Design review of the part shown in the three views and the two pictorial views. Dimensions are in mm from the part's minimum x, y and z. A direction names the side the tool comes from. Round coordinates to 2 decimals unless told otherwise and drop trailing zeros. Order: outer loops, then holes, each group sorted by start corner. A loop starts at its lowest first (then second) coordinate and runs counter-clockwise, first axis right, second up.
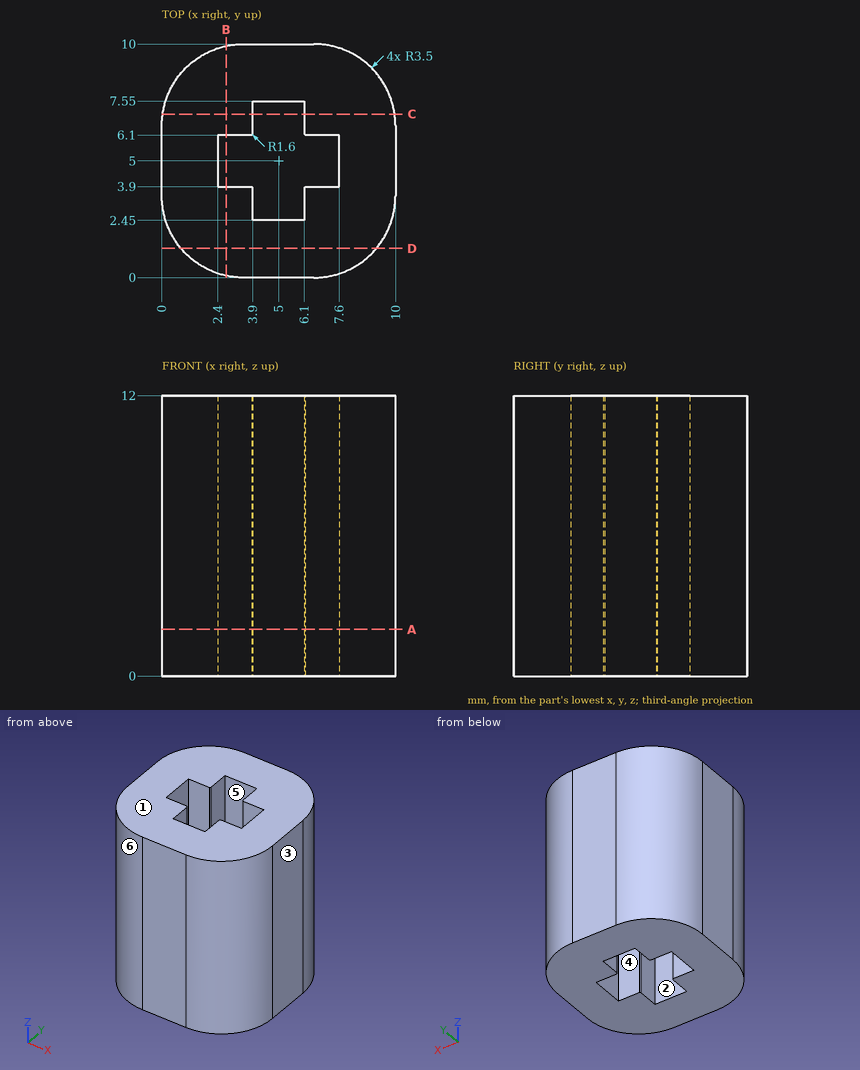
(1) Consider section D-D (y = 1.25). Write out the cut boundary in (x, z), and give its area (3 significant figures).
Data:
outline: (0.82, 0) - (9.18, 0) - (9.18, 12) - (0.82, 12) - close
area: 100 mm2
(2) For the marked faces 5 and 6, list the 3-axis set-ups (+Z, -Z, +X, -X, +Y, -Y) from which the entire face can be reached by the end or side of a thin tool; tool diameter is ignored.
Data:
face 5: +Z, -Z
face 6: +Z, -Z, -X, -Y
(3) Consider section C-C (y = 7). Write out the cut boundary in (x, z).
Data:
outline: (0.04, 0) - (3.9, 0) - (3.9, 12) - (0.04, 12) - close; (6.1, 0) - (9.96, 0) - (9.96, 12) - (6.1, 12) - close
(4) To check wall thickness, follow probe 1 along Y at (x, z) = (6, 3.75); probe 2 along X at (y, z) = (6.5, 10). State the ranges of each line that lie inside material, in increasing order.
Data:
probe 1: y = 0 to 2.45, 7.55 to 10
probe 2: x = 0 to 3.9, 6.1 to 10
(5) Insertion check: pin 1 (3 mm diameter, centred on x = 1.5, z = 10.5, fed in from -Y); pin 2 (0.7 mm diameter, centred on x = 7, z = 8, fed in from +Y). Each pin has a flat end and moves straight along its axis. Give the tip position at first contact, or say it passes through.
Data:
pin 1: stops at y = 0.04
pin 2: stops at y = 10
(6) Consider section A-A (z = 2). Write out the cut boundary in (x, y), and give its area (3 significant figures).
Data:
outline: (0, 3.5) arc R3.5 ccw to (3.5, 0) - (6.5, 0) arc R3.5 ccw to (10, 3.5) - (10, 6.5) arc R3.5 ccw to (6.5, 10) - (3.5, 10) arc R3.5 ccw to (0, 6.5) - close; hole (2.4, 3.9) - (3.84, 3.9) arc R1.6 ccw to (3.9, 3.84) - (3.9, 2.45) - (6.1, 2.45) - (6.1, 3.84) arc R1.6 ccw to (6.16, 3.9) - (7.6, 3.9) - (7.6, 6.1) - (6.16, 6.1) arc R1.6 ccw to (6.1, 6.16) - (6.1, 7.55) - (3.9, 7.55) - (3.9, 6.16) arc R1.6 ccw to (3.84, 6.1) - (2.4, 6.1) - close
area: 71.7 mm2
(7) Draft analysis for pull direction X (two halves, no side actions). For the marked faces 1, 2, 3 and 4, state which applies: pulls with the +X half, pulls with the -X half, needs draft (parallel to the pull), parting line crosses it, or undercut.
Data:
face 1: needs draft
face 2: undercut
face 3: pulls with the +X half
face 4: undercut
(8) Consider section B-B (x = 2.75). Write out the cut boundary in (y, z).
Data:
outline: (0.08, 0) - (3.9, 0) - (3.9, 12) - (0.08, 12) - close; (6.1, 0) - (9.92, 0) - (9.92, 12) - (6.1, 12) - close
